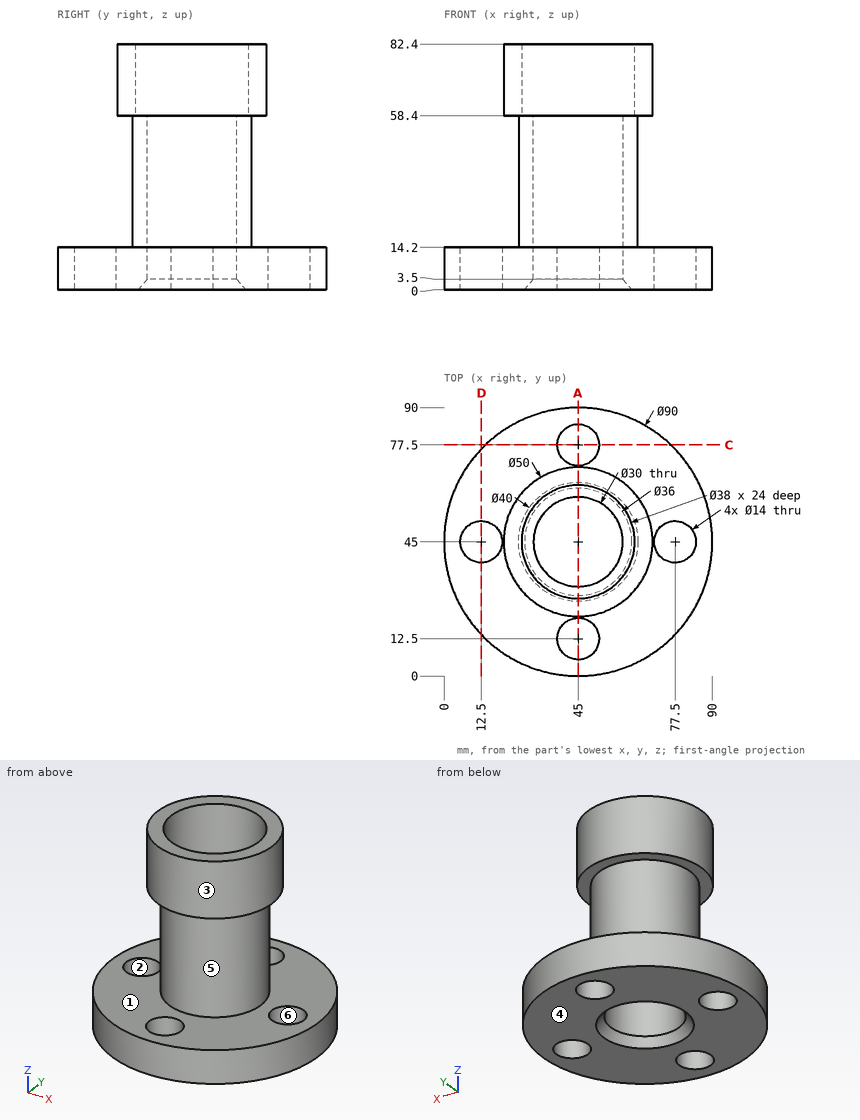
Print and shaded views of the part. All mm, measured from the part's lowest x, y and z. A direction names the side the tool comes from. Coordinates: 2 decimals unless noted, no trailing zeros. Loops run counter-clockwise (first coordinate to the right, second up) from the corner with the lowest first, then second, coordinate; pieces in that order, holes last. Notation, with made-up numbers: (66.25, -31.75) - (122.25, -31.75) arc R29 cw to (122.25, -11.75) - close; hole circle Ø6 at (39.5, 2.25). An arc over 180 degrees is marked (long way). Write item = value, one per line. Start each with the question number.
Item 1: Drop flat-ended pins along their axis: pin 1 Ø10 at (x, z) = (49, 34) entering from -Y; pin 2 Ø24 at (x, y) = (45, 45) entering from -Z; pin 3 Ø22.5 at (x, y) = (45, 77.5) entering from -Z; pin 4 Ø2 at (x, z) = (64, 11.5) entering from -Y. Give the stop position or say it passes through.
Item 2: Pull direction Y, two halves, no side cores. Call the marked faces 4, 5 and 6: +Y half, -Y half, draft (parallel to the pull), parting line (faces both ways), or undercut.
Item 3: Saw through at A-A, the plane x = 45. State how many separate pieces and enclosed holes the cut face has, then the cut area to 3 significant figures.
Item 4: Saw through at C-C, the plane y = 77.5. List the corners of the cut face in (x, z), then the cut area to 3 significant figures.
Item 5: 3-axis set-ups, long thin cutter, end or side, ignore diameter. For the marked faces 1, 2 and 3: which of +Z, -Z, +X, -X, +Y, -Y reach the whole face in a straight line?
Item 6: Wall check: probe 1 along Y at (x, z) = (45, 10); probe 2 along Y at (x, z) = (45, 26); probe 3 along Y at (x, z) = (45, 69). Give the ranges that are in metal, low to high. Write a range as [from, to].
Answers:
q1.pin_1 = 25
q1.pin_2 = through
q1.pin_3 = 0
q1.pin_4 = 3.76
q2.face_4 = draft
q2.face_5 = parting line
q2.face_6 = undercut
q3.separate_pieces = 4
q3.enclosed_holes = 0
q3.area = 1,170 mm2
q4.outline = (13.88, 0) - (38, 0) - (38, 14.2) - (13.88, 14.2) - close; (52, 0) - (76.12, 0) - (76.12, 14.2) - (52, 14.2) - close
q4.area = 685 mm2
q5.face_1 = none
q5.face_2 = +Z, -Z
q5.face_3 = +Z
q6.probe_1 = [0, 5.5], [19.5, 30], [60, 70.5], [84.5, 90]
q6.probe_2 = [25, 30], [60, 65]
q6.probe_3 = [20, 26], [64, 70]
